Source: CAD feature listing. Evaluate the final solid. Frame: model axes, mm. Give positions to 0.01 mm unless a question says otherwise; leave off trailing zeros. Loops run counter-clockwise (first coordinate to the right, second up) from the corner with the lowest first, then second, coordinate; pieces in that order, holes last. Notation, with made-up numbers: M 74,28 L 93,28 A19 cw 93,50 Z; hole C -37,87 d8. An arc over 180 degrees is marked long. Put each result on its own line as item: value.
from build123d import *

# Parameters (mm, degrees)
SKETCH1_W           = 130
SKETCH1_H           = 30
BOSS_EXTRUDE1_DEPTH = 22
SKETCH2_RX          = 15.461746976
SKETCH2_RY          = 5.884694745
CUT_EXTRUDE1_DEPTH  = 75.893257373
SKETCH3_R           = 3
CUT_EXTRUDE2_DEPTH  = 71.242437461
SKETCH4_W           = 1.384926884
SKETCH4_H           = 15.203419573
CUT_EXTRUDE3_DEPTH  = 2


with BuildPart() as part:
    # Sketch1 → Boss-Extrude1 (new body)
    with BuildSketch(Plane(origin=(0, 0, 0), x_dir=(1, 0, 0), z_dir=(0, 1, 0))):
        Rectangle(SKETCH1_W, SKETCH1_H)
    extrude(amount=BOSS_EXTRUDE1_DEPTH)

    # Sketch2 → Cut-Extrude1 (cut, through all)
    with BuildSketch(Plane.XY.offset(15)):
        with Locations((0, 11)):
            Ellipse(SKETCH2_RX, SKETCH2_RY)
    extrude(amount=-CUT_EXTRUDE1_DEPTH, mode=Mode.SUBTRACT)

    # Sketch3 → Cut-Extrude2 (cut, through all)
    with BuildSketch(Plane(origin=(0, 22, 0), x_dir=(1, 0, 0), z_dir=(0, 1, 0))):
        with Locations(Location((-53, 7.5, 0), (0, 0, 270))):
            Circle(SKETCH3_R)
        with Locations(Location((53, 7.5, 0), (0, 0, 90))):
            Circle(SKETCH3_R)
        with Locations(Location((53, -7.5, 0), (0, 0, 270))):
            Circle(SKETCH3_R)
        with Locations(Location((-53, -7.5, 0), (0, 0, 90))):
            Circle(SKETCH3_R)
    extrude(amount=-CUT_EXTRUDE2_DEPTH, mode=Mode.SUBTRACT)

    # Sketch4 → Cut-Extrude3 (cut)
    with BuildSketch(Plane.ZY.offset(65)):
        with Locations((0, 9.722789651)):
            Rectangle(SKETCH4_W, SKETCH4_H)
    extrude(amount=-CUT_EXTRUDE3_DEPTH, mode=Mode.SUBTRACT)


solid = part.part
1. Section query B-B (z = 7.5). State how many separate pieces and enclosed holes the cut face has, plus the area to 3 significant figures.
Found:
separate pieces: 3
enclosed holes: 1
area: 2,310 mm^2
2. Draft query along X for faces 1 (the flat face through (-1, 0, 0)), 2 (the cylindrical face through (-55.53, 11.15, 5.89)), 3 (the flat face through (65, 11, 0)). Return one class per face: pulls with the +X half, pulls with the -X half, needs draft (parallel to the pull), parting line crosses it, or undercut.
Found:
face 1: needs draft
face 2: undercut
face 3: pulls with the +X half
3. Section query A-A (x = -53). Output: boundary loops of the cut face in (y, z).
Found:
outline: M 0,-15 L 22,-15 L 22,-10.5 L 0,-10.5 Z; M 0,-4.5 L 22,-4.5 L 22,4.5 L 0,4.5 Z; M 0,10.5 L 22,10.5 L 22,15 L 0,15 Z
4. Contact query for a flat-ended pin moving along its axis: P1, Ø3.5, axis at x = -53, z = -7.5, coming from the -Y side. Output: stop coordinate, or through.
Found:
P1: through
5. Material intervals for line 1 (X direction, y = 11.25, z = -7.5); line 2 (X direction, y = 17, z = 7.5); line 3 (X direction, y = 11, z = -7.5), sorted ascending. Write a range as from..to.
Found:
line 1: -65..-56, -50..-15.45, 15.45..50, 56..65
line 2: -65..-56, -50..50, 56..65
line 3: -65..-56, -50..-15.46, 15.46..50, 56..65
